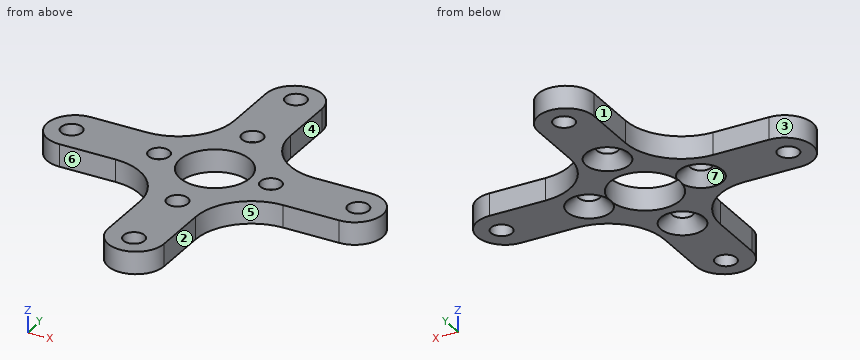
```python
from build123d import *

# Parameters (mm, degrees)
SKETCH_1_R      = 5
SKETCH_1_R_2    = 1.5
EXTRUDE_1_DEPTH = 3.2
CHAMFER_1_SIZE  = 1.6


with BuildPart() as part:
    # Эскиз1 → Бобышка-Вытянуть1 (new body)
    with BuildSketch(Plane.XY):
        with BuildLine():
            Line((-4, 20), (-4, 12))
            ThreePointArc((-4, 12), (-6.343145751, 6.343145751), (-12, 4))
            Line((-12, 4), (-20, 4))
            ThreePointArc((-20, 4), (-24, 0), (-20, -4))
            Line((-20, -4), (-12, -4))
            ThreePointArc((-12, -4), (-6.343145751, -6.343145751), (-4, -12))
            Line((-4, -12), (-4, -20))
            ThreePointArc((-4, -20), (0, -24), (4, -20))
            Line((4, -20), (4, -12))
            ThreePointArc((4, -12), (6.343145751, -6.343145751), (12, -4))
            Line((12, -4), (20, -4))
            ThreePointArc((20, -4), (24, 0), (20, 4))
            Line((20, 4), (12, 4))
            ThreePointArc((12, 4), (6.343145751, 6.343145751), (4, 12))
            Line((4, 12), (4, 20))
            ThreePointArc((4, 20), (0, 24), (-4, 20))
        make_face()
        Circle(SKETCH_1_R, mode=Mode.SUBTRACT)
        with Locations((0, 9.5)):
            Circle(SKETCH_1_R_2, mode=Mode.SUBTRACT)
        with Locations((0, -9.5)):
            Circle(SKETCH_1_R_2, mode=Mode.SUBTRACT)
        with Locations((-8, 0)):
            Circle(SKETCH_1_R_2, mode=Mode.SUBTRACT)
        with Locations((8, 0)):
            Circle(SKETCH_1_R_2, mode=Mode.SUBTRACT)
        with Locations((0, 20.5)):
            Circle(SKETCH_1_R_2, mode=Mode.SUBTRACT)
        with Locations((20.5, 0)):
            Circle(SKETCH_1_R_2, mode=Mode.SUBTRACT)
        with Locations((-20.5, 0)):
            Circle(SKETCH_1_R_2, mode=Mode.SUBTRACT)
        with Locations((0, -20.5)):
            Circle(SKETCH_1_R_2, mode=Mode.SUBTRACT)
    extrude(amount=EXTRUDE_1_DEPTH)

    # Фаска1
    # the kernel refuses this chamfer: 1.6 mm, written as the material it takes off along each edge
    with BuildSketch(Plane(origin=(0, 9.5, 0), x_dir=(1, 0, 0), z_dir=(0, -1, 0))) as chamfer_1_piece_1:
        Polygon((1.5, CHAMFER_1_SIZE), (1.5 + CHAMFER_1_SIZE, 0), (1.5, 0), align=None)
    revolve(axis=Axis((0, 9.5, 0), (0, 0, 1)), mode=Mode.SUBTRACT)
    with BuildSketch(Plane(origin=(0, -9.5, 0), x_dir=(1, 0, 0), z_dir=(0, -1, 0))) as chamfer_1_piece_2:
        Polygon((1.5, CHAMFER_1_SIZE), (1.5 + CHAMFER_1_SIZE, 0), (1.5, 0), align=None)
    revolve(axis=Axis((0, -9.5, 0), (0, 0, 1)), mode=Mode.SUBTRACT)
    with BuildSketch(Plane(origin=(-8, 0, 0), x_dir=(1, 0, 0), z_dir=(0, -1, 0))) as chamfer_1_piece_3:
        Polygon((1.5, CHAMFER_1_SIZE), (1.5 + CHAMFER_1_SIZE, 0), (1.5, 0), align=None)
    revolve(axis=Axis((-8, 0, 0), (0, 0, 1)), mode=Mode.SUBTRACT)
    with BuildSketch(Plane(origin=(8, 0, 0), x_dir=(1, 0, 0), z_dir=(0, -1, 0))) as chamfer_1_piece_4:
        Polygon((1.5, CHAMFER_1_SIZE), (1.5 + CHAMFER_1_SIZE, 0), (1.5, 0), align=None)
    revolve(axis=Axis((8, 0, 0), (0, 0, 1)), mode=Mode.SUBTRACT)


solid = part.part
```
Model file for the job. Use its own axes, mm. Face numbers are marked on the shaded views. A direction names the side the tool comes from. Coordinates: 2 decimals unless noted, no trailing zeros. Loops run counter-clockwise (first coordinate to the right, second up) from the corner with the lowest first, then second, coordinate; pieces in that order, holes last. Notation, with made-up numbers: (34.5, 77.5) -> (65.5, 77.5) arc R33 ccw to (65.5, 113.5) -> close; hole circle Ø2 at (60.25, 76.25). An arc over 180 degrees is marked (long way). Answer as a JSON object with one key per item and string values.
Q1. Cut at B-B (x = -8). List the corners of the cut face in (y, z), and give its area (3 significant figures).
Report:
{"outline": "(-5.07, 0) -> (-3.1, 0) -> (-1.5, 1.6) -> (-1.5, 3.2) -> (-5.07, 3.2) -> close; (1.5, 1.6) -> (3.1, 0) -> (5.07, 0) -> (5.07, 3.2) -> (1.5, 3.2) -> close", "area": "20.3 mm2"}
Q2. Pull direction X, two halves, no side cores. Call the marked faces 5, 6 and 7: released by +X, released by -X, zero draft, split by the parting line, or undercut.
Report:
{"face 5": "released by +X", "face 6": "zero draft", "face 7": "undercut"}
Q3. Cut at C-C (y = 9.5). List the corners of the cut face in (x, z), and give its area (3 significant figures).
Report:
{"outline": "(-4.4, 0) -> (-3.1, 0) -> (-1.5, 1.6) -> (-1.5, 3.2) -> (-4.4, 3.2) -> close; (1.5, 1.6) -> (3.1, 0) -> (4.4, 0) -> (4.4, 3.2) -> (1.5, 3.2) -> close", "area": "16.0 mm2"}
Q4. 3-axis set-ups, long thin cutter, end or side, ignore diameter. For the marked faces 1, 2, 3 and 4: which of +Z, -Z, +X, -X, +Y, -Y reach the whole face in a straight line?
Report:
{"face 1": "+Z, -Z, -X, +Y", "face 2": "+Z, -Z, +X, -Y", "face 3": "+Z, -Z, -X", "face 4": "+Z, -Z, +X, +Y"}
Q5. Cut at A-A (z = 2.35). State how many separate pieces and enclosed holes the cut face has, and give its area (3 significant figures).
Report:
{"separate pieces": "1", "enclosed holes": "9", "area": "596 mm2"}
Q6. Probe probe 1 along Y at (x, z) = (0, 1.7); probe 2 along X at (y, z) = (17, 2.3). List the from-to ranges inside material, lowest first.
Report:
{"probe 1": "y = -24 to -22, -19 to -11, -8 to -5, 5 to 8, 11 to 19, 22 to 24", "probe 2": "x = -4 to 4"}
Q7. Flat gauge pins, fed straight in: P1, Ø1.8, axis at x = 0, y = 9.5, coming from the -Z side; P2, Ø1, axis at x = -16, z = 1.5, coming from the -Y side; P3, Ø4, axis at x = 0, y = -9.5, coming from the -Z side; P4, Ø5, axis at x = -8, y = 0, coming from the -Z side. Where does each tip first touch, or does it go through?
Report:
{"P1": "passes through", "P2": "stops at y = -4", "P3": "stops at z = 1.1", "P4": "stops at z = 0.6"}
